```python
from build123d import *

# Parameters (mm, degrees)
SKETCH1_R           = 12
BOSS_EXTRUDE1_DEPTH = 10
SKETCH2_W           = 32
SKETCH2_H           = 5
BOSS_EXTRUDE2_DEPTH = 25
SKETCH3_R           = 4
CUT_EXTRUDE1_DEPTH  = 25


with BuildPart() as part:
    # Sketch1 → Boss-Extrude1 (new body)
    with BuildSketch(Plane.XY):
        with BuildLine():
            Line((-16, -27.5), (16, -27.5))
            Line((16, -27.5), (16, 25.5))
            ThreePointArc((16, 25.5), (15.414213562, 26.914213562), (14, 27.5))
            Line((14, 27.5), (-14, 27.5))
            ThreePointArc((-14, 27.5), (-15.414213562, 26.914213562), (-16, 25.5))
            Line((-16, 25.5), (-16, -27.5))
        make_face()
        with Locations((0, 9.5)):
            Circle(SKETCH1_R, mode=Mode.SUBTRACT)
    extrude(amount=BOSS_EXTRUDE1_DEPTH)

    # Sketch2 → Boss-Extrude2 (add)
    with BuildSketch(Plane.XY.offset(10)):
        with Locations((0, -25)):
            Rectangle(SKETCH2_W, SKETCH2_H)
    extrude(amount=BOSS_EXTRUDE2_DEPTH)

    # Sketch3 → Cut-Extrude1 (cut)
    with BuildSketch(Plane(origin=(0, -22.5, 0), x_dir=(1, 0, 0), z_dir=(0, 1, 0))):
        with Locations((-7, -22.5)):
            Circle(SKETCH3_R)
        with Locations((7, -22.5)):
            Circle(SKETCH3_R)
    extrude(amount=-CUT_EXTRUDE1_DEPTH, mode=Mode.SUBTRACT)


solid = part.part
```
Geometry: final body of the model. Coordinates: model frame, mm. A direction names the side the tool comes from. Round coordinates to 2 decimals unless told otherwise and drop trailing zeros. Loops run counter-clockwise (first coordinate to the right, second up) from the corner with the lowest first, then second, coordinate; pieces in that order, holes last. Notation, with made-up numbers: (12.5, 89) -> (41.5, 89) arc R17 ccw to (41.5, 99) -> close; hole circle Ø6 at (17, 85.5). An arc over 180 degrees is marked (long way). Use one line per item in the form item = value. Start each with the question number.
1) Draft query along X for faces 3 (the flat face through (0, -3, 10)), 4 (the cylindrical face through (6.479, -24.965, 18.534)), 5 (the cylindrical face through (15.43, 26.9, 4.93)). Return one class per face: released by +X, released by -X, zero draft, split by the parting line, or undercut.
2) Section C-C on y = 9.5. Output: boundary loops of the cut face in (x, z).
3) Line query: L1, parallel to X at y = -25.3, z = 22.5; L2, parallel to Z at x = -7, y = -24; L3, parallel to Y at x = 0, z = 8. Output: solid intervals per line, ascending.
4) Section A-A on z = 4. Output: boundary loops of the cut face in (x, y).
5) First-contact query: P1, Ø8, axis at x = -9, y = 1.5, coming from the +Z side; P2, Ø3, axis at x = -2, y = -8.5, coming from the -Z side. Flat tips, straight axial feed; report the tip coordinate or a pass-through.
6) Access query for faces 1 (the cylindrical face through (-7.521, -24.965, 18.534)), 2 (the flat face through (0, -22.5, 22)). Directions: +Z, -Z, +X, -X, +Y, -Y. A direction counts if a zero-diameter tool reaches every point of the face in a straight line with its end or side. Return the directions, or none.
7) Section B-B on x = 0. Output: boundary loops of the cut face in (y, z), then the cut area to 3 significant figures.
8) Section D-D on z = 22.5. Output: boundary loops of the cut face in (x, y), then the cut area to 3 significant figures.
Response:
q1.face_3 = zero draft
q1.face_4 = undercut
q1.face_5 = released by +X
q2.outline = (-16, 0) -> (-12, 0) -> (-12, 10) -> (-16, 10) -> close; (12, 0) -> (16, 0) -> (16, 10) -> (12, 10) -> close
q3.L1 = -16 to -11, -3 to 3, 11 to 16
q3.L2 = 0 to 18.5, 26.5 to 35
q3.L3 = -27.5 to -2.5, 21.5 to 27.5
q4.outline = (-16, -27.5) -> (16, -27.5) -> (16, 25.5) arc R2 ccw to (14, 27.5) -> (-14, 27.5) arc R2 ccw to (-16, 25.5) -> close; hole circle Ø24 at (0, 9.5)
q5.P1 = 10
q5.P2 = 0
q6.face_1 = +Y, -Y
q6.face_2 = +Z, +X, -X, +Y
q7.outline = (-27.5, 0) -> (-2.5, 0) -> (-2.5, 10) -> (-22.5, 10) -> (-22.5, 35) -> (-27.5, 35) -> close; (21.5, 0) -> (27.5, 0) -> (27.5, 10) -> (21.5, 10) -> close
q7.area = 435 mm^2
q8.outline = (-16, -27.5) -> (-11, -27.5) -> (-11, -22.5) -> (-16, -22.5) -> close; (-3, -27.5) -> (3, -27.5) -> (3, -22.5) -> (-3, -22.5) -> close; (11, -27.5) -> (16, -27.5) -> (16, -22.5) -> (11, -22.5) -> close
q8.area = 80.0 mm^2
